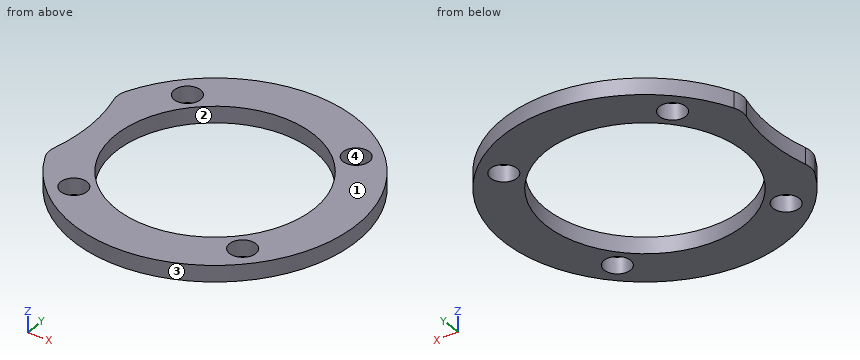
```python
from build123d import *

# Parameters (mm, degrees)
SKETCH_1_R          = 18.25
SKETCH_1_R_2        = 12.75
EXTRUDE_1_DEPTH     = 1.05
SKETCH_2_R          = 22
CUT_EXTRUDE_1_DEPTH = 21.05
SKETCH_3_R          = 1.7
CUT_EXTRUDE_2_DEPTH = 16.05
FILLET_1_R          = 3


with BuildPart() as part:
    # 草图1 → 凸台-拉伸1 (new, symmetric)
    with BuildSketch(Plane.XY):
        Circle(SKETCH_1_R)
        Circle(SKETCH_1_R_2, mode=Mode.SUBTRACT)
    extrude(amount=EXTRUDE_1_DEPTH, both=True)

    # 草图2 → 切除-拉伸1 (cut, symmetric)
    with BuildSketch(Plane.XY.offset(1.05)):
        with Locations((-38, 0)):
            Circle(SKETCH_2_R)
    extrude(amount=CUT_EXTRUDE_1_DEPTH, both=True, mode=Mode.SUBTRACT)

    # 草图3 → 切除-拉伸2 (cut, symmetric)
    with BuildSketch(Plane.XY.offset(1.05)):
        with Locations((10.783378413, 10.783378413)):
            Circle(SKETCH_3_R)
        with Locations((10.783378413, -10.783378413)):
            Circle(SKETCH_3_R)
        with Locations((-10.783378413, -10.783378413)):
            Circle(SKETCH_3_R)
        with Locations((-10.783378413, 10.783378413)):
            Circle(SKETCH_3_R)
    extrude(amount=CUT_EXTRUDE_2_DEPTH, both=True, mode=Mode.SUBTRACT)

    # 圆角1
    fillet_1_edges = [part.edges().sort_by_distance(p)[0] for p in [
        (-17.013980263, -6.60204329, 0),
        (-17.013980263, 6.60204329, 0),
    ]]
    fillet(fillet_1_edges, radius=FILLET_1_R)


solid = part.part
```
Work out the finished part from the listing and answer in its coordinate system (mm). Face numbers are marked on the shaded views. Coordinates: 2 decimals unless noted, no trailing zeros. Loops run counter-clockwise (first coordinate to the right, second up) from the corner with the lowest first, then second, coordinate; pieces in that order, holes last. Notation, with made-up numbers: (38.5, 11) - (65.5, 11) arc R20 ccw to (65.5, 42) - close; hole circle Ø5 at (-28.75, 3). An arc over 180 degrees is marked (long way). Use a Markdown table: item, result.
Item 1: Find section D-D, the plane z = 0.4. State how many separate pieces and enclosed holes the cut face has, and give its area (3 significant figures).
Evaluation:
| item | result |
|---|---|
| separate pieces | 1 |
| enclosed holes | 5 |
| area | 479 mm2 |
Item 2: Consider probe 1 along Y at (x, z) = (0.5, 0.5); probe 2 along X at (y, z) = (10, -0.6); probe 3 along X at (y, z) = (-5, 0.2). Determine where each line is inside the solid, lowest interval first. Write a range as from..to.
Evaluation:
| item | result |
|---|---|
| probe 1 | y = -18.24..-12.74, 12.74..18.24 |
| probe 2 | x = -15.27..-12.29, -9.27..-7.91, 7.91..9.27, 12.29..15.27 |
| probe 3 | x = -16.58..-11.73, 11.73..17.55 |
Item 3: Given pin 1 Ø4 at (x, y) = (-9, -3.5) entering from +Z; pin 2 Ø1 at (x, z) = (3.5, -0.5) entering from +Y, each flat-ended and moving along its own axis, determine where each tip first touches the part or whether it passes through.
Evaluation:
| item | result |
|---|---|
| pin 1 | passes through |
| pin 2 | stops at y = 18 |
Item 4: Find section A-A, the plane y = 0. Determine the outline of the cut face in (x, z), and give its area (3 significant figures).
Evaluation:
| item | result |
|---|---|
| outline | (-16, -1.05) - (-12.75, -1.05) - (-12.75, 1.05) - (-16, 1.05) - close; (12.75, -1.05) - (18.25, -1.05) - (18.25, 1.05) - (12.75, 1.05) - close |
| area | 18.4 mm2 |
Item 5: The mould has two halves that part along X. Classify the marked faces 1, 2, 3 and 4: +X half, -X half, draft (parallel to the pull), parting line (faces both ways), or undercut.
Evaluation:
| item | result |
|---|---|
| face 1 | draft |
| face 2 | undercut |
| face 3 | parting line |
| face 4 | undercut |
Item 6: Find section C-C, the plane y = 12. Determine the outline of the cut face in (x, z), and give its area (3 significant figures).
Evaluation:
| item | result |
|---|---|
| outline | (-13.75, -1.05) - (-11.97, -1.05) - (-11.97, 1.05) - (-13.75, 1.05) - close; (-9.6, -1.05) - (-4.31, -1.05) - (-4.31, 1.05) - (-9.6, 1.05) - close; (4.31, -1.05) - (9.6, -1.05) - (9.6, 1.05) - (4.31, 1.05) - close; (11.97, -1.05) - (13.75, -1.05) - (13.75, 1.05) - (11.97, 1.05) - close |
| area | 29.7 mm2 |
Item 7: Find section B-B, the plane x = 0. Determine the outline of the cut face in (y, z).
Evaluation:
| item | result |
|---|---|
| outline | (-18.25, -1.05) - (-12.75, -1.05) - (-12.75, 1.05) - (-18.25, 1.05) - close; (12.75, -1.05) - (18.25, -1.05) - (18.25, 1.05) - (12.75, 1.05) - close |
